Can you work these out from the model? Positions are in its coordinate system, mm. Coordinates: 2 decimals unless noted, no trailing zeros. Order: outer loops, then holes, each group sorted by start corner. A loop starts at its lowest first (then second) coordinate and runs counter-clockwise, first axis right, second up. Notation, with made-up numbers: (69, 84) -> (108, 84) arc R19 cw to (108, 110) -> close; hole circle Ø11 at (11, 76.25). An arc over 180 degrees is marked (long way). Answer in a Markdown table with one row per item. Add a question column.
1. Imagine slicing it at A-A on x = 1.3. Write out the boundary of the cut face in (y, z).
2. If I drill on line 1 along X through (y, z) = (-14.5, 17.5); line 2 along Y through (x, z) = (-2.1, 1.75); line 3 along Y through (x, z) = (0.2, 7.75) (3 decimals), over which ranges is the centre line in solid material (lowest first)? Write a range as [from, to].
3. Imagine slicing it at B-B on y = -15. Write out the boundary of the cut face in (x, z), plus the area to 3 significant figures.
4. We'd pull the mould along Y, two halves only. Please class faces 1 (the face through (0, -1, 9.4)), 2 (the face through (-0.036, -15.838, 9.658)), 3 (the face through (0, -7, 19.05)): pulls with the +Y half, pulls with the -Y half, needs draft (parallel to the pull), parting line crosses it, or undercut.
5. Will this pin go through, and if not, where does the flat tip stop? pin 1 (1.5 mm diameter, centred on x = 1, z = 13, fed in from +Y).
from build123d import *

# Parameters (mm, degrees)
ESQUISSE1_W             = 5.08
ESQUISSE1_H             = 19.05
BOSS_EXTRU_1_DEPTH      = 20.828
ENL_V_MAT_EXTRU_1_DEPTH = 6.08
ENL_V_MAT_EXTRU_2_DEPTH = 20.05


with BuildPart() as part:
    # Esquisse1 → Boss.-Extru.1 (new body)
    with BuildSketch(Plane(origin=(0, 0, 0), x_dir=(1, 0, 0), z_dir=(0, 1, 0))):
        with Locations((0, -9.525)):
            Rectangle(ESQUISSE1_W, ESQUISSE1_H)
    extrude(amount=-BOSS_EXTRU_1_DEPTH)

    # Esquisse2 → Enlèv. mat.-Extru.1 (cut, through all)
    with BuildSketch(Plane(origin=(2.54, 0, 0), x_dir=(0, 0, -1), z_dir=(1, 0, 0))):
        Polygon((0, -1.971986417), (-19.05, 0), (0, 0), align=None)
    extrude(amount=-ENL_V_MAT_EXTRU_1_DEPTH, mode=Mode.SUBTRACT)

    # Esquisse3 → Enlèv. mat.-Extru.2 (cut, through all)
    with BuildSketch(Plane.XY.offset(19.05)):
        Polygon((-2.54, -20.828), (-2.54, -13.208), (2.54, -18.542), (2.54, -20.828), align=None)
    extrude(amount=-ENL_V_MAT_EXTRU_2_DEPTH, mode=Mode.SUBTRACT)


solid = part.part
Answers follow:
| question | item | result |
|---|---|---|
| 1 | outline | (-17.24, 0) -> (-1.97, 0) -> (0, 19.05) -> (-17.24, 19.05) -> close |
| 2 | line 1 | x = [-1.31, 2.54] |
| 2 | line 2 | y = [-13.67, -1.79] |
| 2 | line 3 | y = [-16.085, -1.17] |
| 3 | outline | (-0.83, 0) -> (2.54, 0) -> (2.54, 19.05) -> (-0.83, 19.05) -> close |
| 3 | area | 64.3 mm² |
| 4 | face 1 | pulls with the +Y half |
| 4 | face 2 | pulls with the -Y half |
| 4 | face 3 | needs draft |
| 5 | pin 1 | stops at y = -0.55 |
